Here's how the part is built. I have some questions about the finished solid (model axes, mm). Face numbers are marked on the shaded views. Coordinates: 2 decimals unless noted, no trailing zeros. Write each loop counter-clockwise with the first axis right and the second up, starting at its lowest first coordinate (ties: lowest second). Pieces come first, ordered by that corner, then holes.
(1) Imagine slicing it at B-B, the plane z = -9.5. List the corners of the cut face in (x, y) for me.
(2) For pin 1 Ø1.5 at (y, z) = (1, -4.5) entering from -X; pin 2 Ø0.8 at (y, z) = (2, -3) entering from -X; pin 3 Ø0.9 at (x, y) = (-11, 1) entering from +Z, each with a flat end and sliding along its axis, tell me the tip position at first contact or that it passes through.
(3) Imagine slicing it at C-C, the plane y = 2.4. List the corners of the cut face in (x, z) for me.
(4) Imagine slicing it at D-D, the plane x = -17. List the corners of the cut face in (y, z) for me, plus the area to 3 significant figures.
(5) Please list where these lines run through material, in increasing order: probe 1 along X at (y, z) = (2, -9.5); probe 2 along X at (y, z) = (2.45, -12.25); probe 3 along X at (y, z) = (2.1, -6.25).
(6) Imagine slicing it at A-A, the plane x = -38.5. List the corners of the cut face in (y, z) for me, plus the area to 3 significant figures.
(7) Thinking about a two-plate mould opening in Y: for the marked faces 1 and 2, which applies, released by +Y, released by -Y, zero draft, split by the parting line, or undercut?
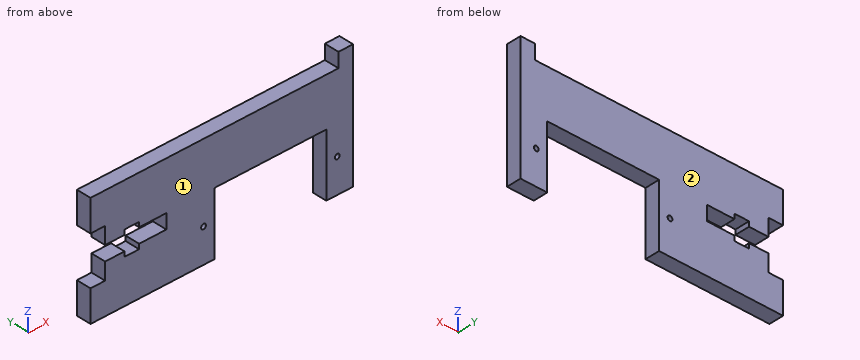
```python
from build123d import *

# Parameters (mm, degrees)
SKETCH_1_R      = 0.5
EXTRUDE_1_DEPTH = 3


with BuildPart() as part:
    # 草图1 → 凸台-拉伸1 (new body)
    with BuildSketch(Plane(origin=(0, 0, 0), x_dir=(1, 0, 0), z_dir=(0, 1, 0))):
        Polygon((-45.982728377, 0), (-45.982728377, -6.5), (5.017271623, -6.5), (5.017271623, -9.5), (8.017271623, -9.5), (8.017271623, 16.5), (2.517271623, 16.5), (2.517271623, 3.5), (-20.482728377, 3.5), (-20.482728377, 16.5), (-45.982728377, 16.5), (-45.982728377, 10), (-42.982728377, 10), (-42.982728377, 6.5), (-38.982728377, 6.5), (-38.982728377, 7.5), (-35.982728377, 7.5), (-35.982728377, 6.5), (-30.382728377, 6.5), (-30.382728377, 3.5), (-35.982728377, 3.5), (-35.982728377, 2.5), (-38.982728377, 2.5), (-38.982728377, 3.5), (-42.982728377, 3.5), (-42.982728377, 0), align=None)
        with Locations(Location((-22.732728377, 9.5, 0), (0, 0, 270))):
            Circle(SKETCH_1_R, mode=Mode.SUBTRACT)
        with Locations(Location((4.767271623, 9.5, 0), (0, 0, 270))):
            Circle(SKETCH_1_R, mode=Mode.SUBTRACT)
    extrude(amount=EXTRUDE_1_DEPTH)


solid = part.part
```
Recorded:
1. outline: (-42.98, 0) - (-23.23, 0) - (-23.23, 3) - (-42.98, 3) - close; (-22.23, 0) - (-20.48, 0) - (-20.48, 3) - (-22.23, 3) - close; (2.52, 0) - (4.27, 0) - (4.27, 3) - (2.52, 3) - close; (5.27, 0) - (8.02, 0) - (8.02, 3) - (5.27, 3) - close
2. pin 1: stops at x = -30.38
2. pin 2: stops at x = -42.98
2. pin 3: stops at z = 6.5
3. outline: (-45.98, -16.5) - (-20.48, -16.5) - (-20.48, -3.5) - (2.52, -3.5) - (2.52, -16.5) - (8.02, -16.5) - (8.02, 9.5) - (5.02, 9.5) - (5.02, 6.5) - (-45.98, 6.5) - (-45.98, 0) - (-42.98, 0) - (-42.98, -3.5) - (-38.98, -3.5) - (-38.98, -2.5) - (-35.98, -2.5) - (-35.98, -3.5) - (-30.38, -3.5) - (-30.38, -6.5) - (-35.98, -6.5) - (-35.98, -7.5) - (-38.98, -7.5) - (-38.98, -6.5) - (-42.98, -6.5) - (-42.98, -10) - (-45.98, -10) - close; hole circle Ø1 at (-22.73, -9.5); hole circle Ø1 at (4.77, -9.5)
4. outline: (0, -3.5) - (3, -3.5) - (3, 6.5) - (0, 6.5) - close
4. area: 30.0 mm2
5. probe 1: x = -42.98 to -23.23, -22.23 to -20.48, 2.52 to 4.27, 5.27 to 8.02
5. probe 2: x = -45.98 to -20.48, 2.52 to 8.02
5. probe 3: x = -30.38 to -20.48, 2.52 to 8.02
6. outline: (0, -16.5) - (3, -16.5) - (3, -7.5) - (0, -7.5) - close; (0, -2.5) - (3, -2.5) - (3, 6.5) - (0, 6.5) - close
6. area: 54.0 mm2
7. face 1: released by -Y
7. face 2: released by +Y
